```python
from build123d import *

# Parameters (mm, degrees)
SKETCH1_W           = 240
SKETCH1_H           = 160
BOSS_EXTRUDE1_DEPTH = 5
SKETCH2_R           = 1.6
CUT_EXTRUDE1_DEPTH  = 5
FILLET1_R           = 6


with BuildPart() as part:
    # Sketch1 → Boss-Extrude1 (new body)
    with BuildSketch(Plane(origin=(0, 0, 0), x_dir=(1, 0, 0), z_dir=(0, 1, 0))):
        Rectangle(SKETCH1_W, SKETCH1_H)
    extrude(amount=BOSS_EXTRUDE1_DEPTH)

    # Sketch2 → Cut-Extrude1 (cut)
    with BuildSketch(Plane(origin=(0, 5, 0), x_dir=(1, 0, 0), z_dir=(0, 1, 0))):
        with Locations((-112, 72)):
            Circle(SKETCH2_R)
        with Locations((-112, -72)):
            Circle(SKETCH2_R)
        with Locations((112, 72)):
            Circle(SKETCH2_R)
        with Locations((112, -72)):
            Circle(SKETCH2_R)
        with Locations((10.28, 63.5)):
            Circle(SKETCH2_R)
        with Locations((101.72, 63.5)):
            Circle(SKETCH2_R)
        with Locations((101.72, -63.5)):
            Circle(SKETCH2_R)
        with Locations((10.28, -63.5)):
            Circle(SKETCH2_R)
        with BuildLine():
            Line((-94.3, 30.4), (-94.3, 24))
            ThreePointArc((-94.3, 24), (-92.7, 22.4), (-91.1, 24))
            Line((-91.1, 24), (-91.1, 30.4))
            ThreePointArc((-91.1, 30.4), (-92.7, 32), (-94.3, 30.4))
        make_face()
        with BuildLine():
            Line((-94.3, 12.4), (-94.3, 6))
            ThreePointArc((-94.3, 6), (-92.7, 4.4), (-91.1, 6))
            Line((-91.1, 6), (-91.1, 12.4))
            ThreePointArc((-91.1, 12.4), (-92.7, 14), (-94.3, 12.4))
        make_face()
        with BuildLine():
            Line((-20.9, 12.4), (-20.9, 6))
            ThreePointArc((-20.9, 6), (-19.3, 4.4), (-17.7, 6))
            Line((-17.7, 6), (-17.7, 12.4))
            ThreePointArc((-17.7, 12.4), (-19.3, 14), (-20.9, 12.4))
        make_face()
        with BuildLine():
            Line((-20.9, 30.4), (-20.9, 24))
            ThreePointArc((-20.9, 24), (-19.3, 22.4), (-17.7, 24))
            Line((-17.7, 24), (-17.7, 30.4))
            ThreePointArc((-17.7, 30.4), (-19.3, 32), (-20.9, 30.4))
        make_face()
        with BuildLine():
            Line((-94.3, -62.4), (-94.3, -56))
            ThreePointArc((-94.3, -56), (-92.7, -54.4), (-91.1, -56))
            Line((-91.1, -56), (-91.1, -62.4))
            ThreePointArc((-91.1, -62.4), (-92.7, -64), (-94.3, -62.4))
        make_face()
        with BuildLine():
            Line((-91.1, -44.4), (-91.1, -38))
            ThreePointArc((-91.1, -38), (-92.7, -36.4), (-94.3, -38))
            Line((-94.3, -38), (-94.3, -44.4))
            ThreePointArc((-94.3, -44.4), (-92.7, -46), (-91.1, -44.4))
        make_face()
        with BuildLine():
            Line((-78.5, 55.4), (-33.5, 55.4))
            ThreePointArc((-33.5, 55.4), (-30.9, 58), (-33.5, 60.6))
            Line((-33.5, 60.6), (-78.5, 60.6))
            ThreePointArc((-78.5, 60.6), (-81.1, 58), (-78.5, 55.4))
        make_face()
        with BuildLine():
            Line((-17.7, -62.4), (-17.7, -56))
            ThreePointArc((-17.7, -56), (-19.3, -54.4), (-20.9, -56))
            Line((-20.9, -56), (-20.9, -62.4))
            ThreePointArc((-20.9, -62.4), (-19.3, -64), (-17.7, -62.4))
        make_face()
        with BuildLine():
            Line((-20.9, -44.4), (-20.9, -38))
            ThreePointArc((-20.9, -38), (-19.3, -36.4), (-17.7, -38))
            Line((-17.7, -38), (-17.7, -44.4))
            ThreePointArc((-17.7, -44.4), (-19.3, -46), (-20.9, -44.4))
        make_face()
    extrude(amount=-CUT_EXTRUDE1_DEPTH, mode=Mode.SUBTRACT)

    # Fillet1
    fillet1_edges = [part.edges().sort_by_distance(p)[0] for p in [
        (120, 2.5, 80),
        (-120, 2.5, 80),
        (-120, 2.5, -80),
        (120, 2.5, -80),
    ]]
    fillet(fillet1_edges, radius=FILLET1_R)


solid = part.part
```
Design review of the part built by this model. Coordinates are the model's own, in mm. A direction names the side the tool comes from. Coordinates: 2 decimals unless noted, no trailing zeros. Order: outer loops, then holes, each group sorted by start corner. A loop starts at its lowest first (then second) coordinate and runs counter-clockwise, first axis right, second up.
1) Take a section at B-B, the plane z = -58. Give the boundary of the cut face in (x, y).
2) Take a section at A-A, the plane x = -52. Give the boundary of the cut face in (y, z), and give its area (3 significant figures).
3) Wall thickness on line 1 along X through (y, z) = (4, 60); line 2 along X through (y, z) = (2.5, 72); line 3 along Z through (x, y) = (-93, 3.9): over which ranges is each line inside the solid? List them lowest first.
4) Take a section at C-C, the plane y = 1.7. State how many separate pieces and enclosed holes the cut face has, and give its area (3 significant figures).
5) For faces 1 (the flat face through (120, 2, 1)), 2 (the flat face through (-91.1, 3, -27)), list the 3-axis set-ups (+Z, -Z, +X, -X, +Y, -Y) from which the entire face can be reached by the end or side of a thin tool; tool diameter is ignored.
6) Mouldability with a two-part tool opening along Z and no side actions: class faces 3 (the flat face through (-120, 2, 1)), 4 (the flat face through (-94.3, 3, 41)), 5 (the flat face through (-2, 2, -80)) as +Z half, -Z half, draft (parallel to the pull), parting line (faces both ways), or undercut.
Returned:
1. outline: (-120, 0) - (-81.1, 0) - (-81.1, 5) - (-120, 5) - close; (-30.9, 0) - (120, 0) - (120, 5) - (-30.9, 5) - close
2. outline: (0, -80) - (5, -80) - (5, -60.6) - (0, -60.6) - close; (0, -55.4) - (5, -55.4) - (5, 80) - (0, 80) - close
2. area: 774 mm2
3. line 1: x = -120 to -94.3, -91.1 to -20.9, -17.7 to 120
3. line 2: x = -120 to -113.6, -110.4 to 110.4, 113.6 to 120
3. line 3: z = -80 to -31.97, -22.43 to -13.97, -4.43 to 36.43, 45.97 to 54.43, 63.97 to 80
4. separate pieces: 1
4. enclosed holes: 17
4. area: 37,800 mm2
5. face 1: +Z, -Z, +X, +Y, -Y
5. face 2: +Y, -Y
6. face 3: draft
6. face 4: undercut
6. face 5: -Z half
